from build123d import *

# Parameters (mm, degrees)
F1_DEPTH = 23.67751


with BuildPart() as f1:
    # F0 (on Front) → F1 (new body)
    with BuildSketch(Plane.XZ):
        with BuildLine():
            Line((-71.815483, 52.379653), (-71.815483, 0))
            Line((-71.815483, 0), (0, 0))
            Line((0, 0), (0, 77.384859))
            ThreePointArc((0, 77.384859), (-5.48468, 75.305304), (-8.211866, 70.112161))
            Line((-8.211866, 70.112161), (-11.343726, 70.112161))
            Line((-11.343726, 70.112161), (-11.343726, 67.48306))
            ThreePointArc((-11.343726, 67.48306), (-18.710491, 63.14941), (-27.123494, 61.64239))
            Line((-27.123494, 61.64239), (-28.187953, 61.64239))
            Line((-28.187953, 61.64239), (-28.187953, 58.809962))
            Line((-28.187953, 58.809962), (-37.14551, 58.809962))
            Line((-37.14551, 58.809962), (-37.14551, 52.379653))
            Line((-37.14551, 52.379653), (-71.815483, 52.379653))
        make_face()
    extrude(amount=-F1_DEPTH)

    # F2: F1 across plane


with BuildPart() as f1_1:
    add(f1.part)
    add(f1.part.mirror(Plane.YZ))


solid = f1_1.part
Geometry check sheet. Reference: the model listing, model coordinates, mm. A direction names the side the tool comes from. Coordinates: 2 decimals unless noted, no trailing zeros. Loops run counter-clockwise (first coordinate to the right, second up) from the corner with the lowest first, then second, coordinate; pieces in that order, holes last. Notation, with made-up numbers: (68.25, -9.75) - (101.25, -9.75) arc R23 cw to (101.25, 15.25) - close; hole circle Ø5 at (85, -16.75). An arc over 180 degrees is marked (long way). Use one line per item in the form item = value. Start each with the question number.
Item 1: Section check B-B, the plane x = -32. Enter the section's corners in (y, z), and give its area (3 significant figures).
Item 2: Gauge pin test, flat ends, axial feed: pin 1 (0.9 mm diameter, centred on x = -9, y = 13.5, fed in from +Z); pin 2 (5 mm diameter, centred on x = 53.5, y = 12.5, fed in from +Z); pin 3 (1.9 mm diameter, centred on y = 16.5, z = 57, fed in from -X). Record the tip position at first contact, or that the pin passes through.
Item 3: Thickness scan on probe 1 along Z at (x, y) = (-35, 2); probe 2 along Z at (x, y) = (-47, 19.75); probe 3 along X at (y, z) = (13.75, 59). Record the ranges inside material, lowest first.
Item 4: Section check C-C, the plane x = 47.5. Enter the section's corners in (y, z).
Item 5: Section check A-A, the plane y = 12.75. Enter the section's corners in (x, z), and give its area (3 significant figures).
Item 6: Tool access check on faces 1 (the face through (1, 0, 31)), 2 (the face through (54, 12, 52.38)), 3 (the face through (-10, 12, 70.112)). Record the directions out of +Z, -Z, +X, -X, +Y, -Y that give a thin tool (end or side, any length) a straight path to the whole face; none if there is none.
Computed:
q1.outline = (0, 0) - (23.68, 0) - (23.68, 58.81) - (0, 58.81) - close
q1.area = 1,390 mm2
q2.pin_1 = 70.11
q2.pin_2 = 52.38
q2.pin_3 = -37.15
q3.probe_1 = 0 to 58.81
q3.probe_2 = 0 to 52.38
q3.probe_3 = -28.19 to 28.19
q4.outline = (0, 0) - (23.68, 0) - (23.68, 52.38) - (0, 52.38) - close
q5.outline = (-71.82, 0) - (71.82, 0) - (71.82, 52.38) - (37.15, 52.38) - (37.15, 58.81) - (28.19, 58.81) - (28.19, 61.64) - (27.12, 61.64) arc R24.24 cw to (11.34, 67.48) - (11.34, 70.11) - (8.21, 70.11) arc R8.27 ccw to (-8.21, 70.11) - (-11.34, 70.11) - (-11.34, 67.48) arc R24.24 cw to (-27.12, 61.64) - (-28.19, 61.64) - (-28.19, 58.81) - (-37.15, 58.81) - (-37.15, 52.38) - (-71.82, 52.38) - close
q5.area = 8,500 mm2
q6.face_1 = +Z, -Z, +X, -X, -Y
q6.face_2 = +Z, +X, +Y, -Y
q6.face_3 = +Z, -X, +Y, -Y
